Study the drawing (mm; zero at the part's minimum x, y, z) and answer. A direction names the side the tool comes from. Coordinates: 2 decimals unless noted, no trailing zeros. Order: outer loops, then holes, each group sorted by start corner. A loop starts at its lowest first (then second) coordinate and runs counter-clockwise, first axis right, second up. Notation, with made-up numbers: (10.5, 59) -> (34.5, 59) arc R25 cw to (34.5, 85) -> close; hole circle Ø4 at (-30.5, 0). An arc over 180 degrees is marked (long way). One line per question, with ' | ' between items.
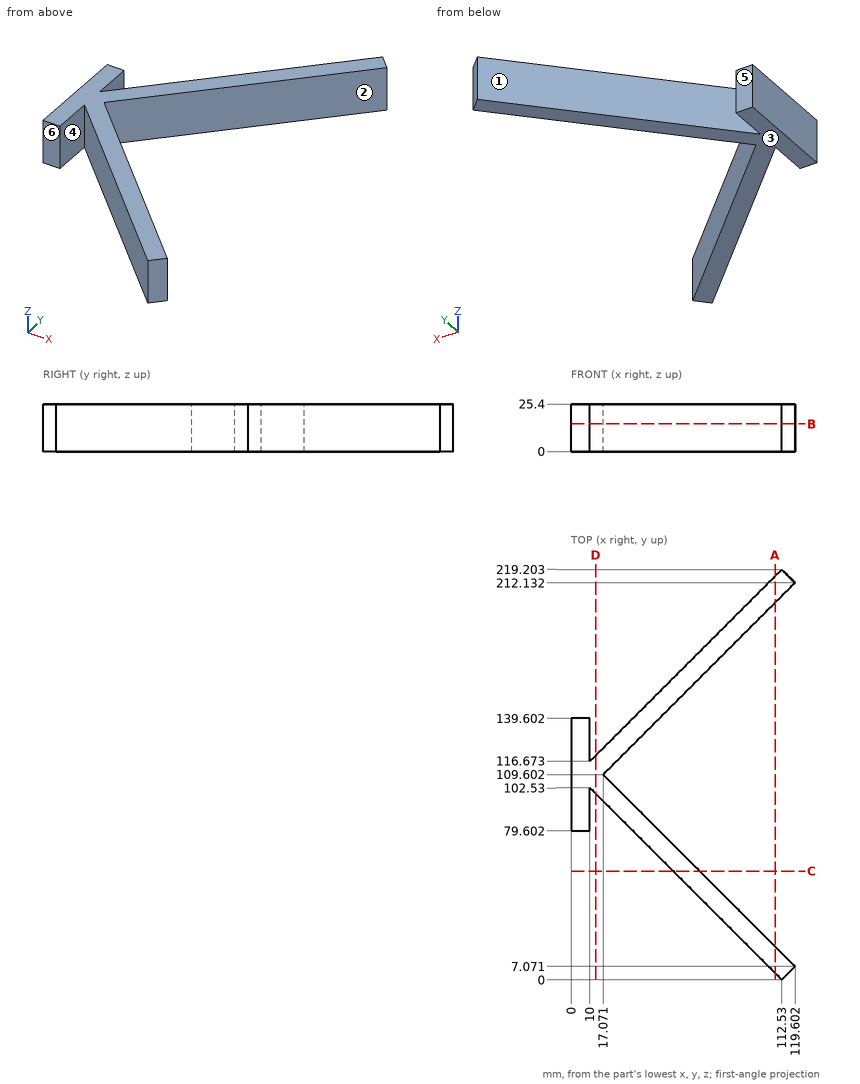
Item 1: Find the intervals of material crossed by L1, parallel to Y at x = 46.5, z = 10.25 (1 decimal); L2, parallel to Y at x = 38.5, z = 6.25 (1 decimal); L3, parallel to X at y = 137.5, z = 5.75 (1 decimal), in increasing order.
Computed values:
L1: y = 66 to 80.2, 139 to 153.2 | L2: y = 74 to 88.2, 131 to 145.2 | L3: x = 0 to 10, 30.8 to 45
Item 2: Section A-A, the plane x = 109 is taken. Give the vertices of the cut face in (y, z).
Computed values:
outline: (3.53, 0) -> (17.67, 0) -> (17.67, 25.4) -> (3.53, 25.4) -> close; (201.53, 0) -> (215.67, 0) -> (215.67, 25.4) -> (201.53, 25.4) -> close
Item 3: Determine the mould class of the marked faces 1, 2 and 3 for opening direction Y: pulls with the +Y half, pulls with the -Y half, needs draft (parallel to the pull), parting line crosses it, or undercut.
Computed values:
face 1: pulls with the +Y half | face 2: undercut | face 3: needs draft
Item 4: Section B-B, the plane z = 14.75 is taken. Give the vertices of the cut face in (x, y), plus the area to 3 significant figures.
Computed values:
outline: (0, 79.6) -> (10, 79.6) -> (10, 102.53) -> (112.53, 0) -> (119.6, 7.07) -> (17.07, 109.6) -> (119.6, 212.13) -> (112.53, 219.2) -> (10, 116.67) -> (10, 139.6) -> (0, 139.6) -> close | area: 3,550 mm^2
Item 5: Section D-D, the plane x = 13 is taken. Give the vertices of the cut face in (y, z), plus the area to 3 significant figures.
Computed values:
outline: (99.53, 0) -> (119.67, 0) -> (119.67, 25.4) -> (99.53, 25.4) -> close | area: 512 mm^2
Item 6: For the marked faces 4, 5 and 6, determine the directions among +Z, -Z, +X, -X, +Y, -Y from which every point of the face is accessible in a straight line to the end or side of a thin tool.
Computed values:
face 4: +Z, -Z, -Y | face 5: +Z, -Z, -X, +Y | face 6: +Z, -Z, -X, -Y
Item 7: Each of these flat-tipped pins is pushed along its axis until it touches: pin 1 Ø5 at (x, z) = (6.5, 11) entering from +Y; pin 2 Ø6 at (x, z) = (60.5, 15) entering from +Y; pin 3 Ø5 at (y, z) = (64, 11.5) entering from -X. Where does it stop, or does it pass through?
Computed values:
pin 1: stops at y = 139.6 | pin 2: stops at y = 170.17 | pin 3: stops at x = 46.03
Item 8: Section C-C, the plane y = 58 is taken. Give the vertices of the cut face in (x, z).
Computed values:
outline: (54.53, 0) -> (68.67, 0) -> (68.67, 25.4) -> (54.53, 25.4) -> close
